Check sheet for the modelled part. Datum: model origin and axes. Units: mm. A direction names the side the tool comes from. Round coordinates to 2 decimals unless told otherwise and drop trailing zeros. Loops run counter-clockwise (first coordinate to the right, second up) from the corner with the lowest first, then second, coordinate; pieces in that order, holes last. Notation, with made-up numbers: (49.25, 27.5) -> (78.25, 27.5) arc R18 cw to (78.25, 36.5) -> close; hole circle Ø7 at (4.5, 61). An arc over 180 degrees is marked (long way). Return JSON: item names as keys, results as strings.
from build123d import *

# Parameters (mm, degrees)
F1_DEPTH        = 5
F2_R            = 22.75
F3_DEPTH        = 1
F5_DEPTH        = 4
F6_DEPTH        = 3
F7_R            = 9
F8_DEPTH        = 4.001
F9_R            = 3
F10_R           = 1
F11_R           = 0.5
F13_D           = 2.75
F13_CBORE_D     = 4.6
F13_CBORE_DEPTH = 2
F14_R           = 1.99999
F15_SIZE        = 0.4
F16_ANGLE       = 180


# Not quite as in the source:
# - a fillet or chamfer is up to 0.001 mm smaller than in the source, because OpenCascade refuses the exact size


with BuildPart() as f1:
    # F0 (on Top) → F1 (new body)
    with BuildSketch(Plane.XY):
        Polygon((23.5, -23.5), (23.5, 23.5), (-23.5, 23.5), (-23.5, 12.5), (-33.5, 12.5), (-33.5, -12.5), (-23.5, -12.5), (-23.5, -23.5), (-12.5, -23.5), (-12.5, -33.5), (12.5, -33.5), (12.5, -23.5), align=None)
    extrude(amount=F1_DEPTH)

    # F2 (on face) → F3 (cut)
    with BuildSketch(Plane(origin=(0, 0, 0), x_dir=(1, 0, 0), z_dir=(0, 0, -1))):
        Circle(F2_R)
    extrude(amount=-F3_DEPTH, mode=Mode.SUBTRACT)

    # F4 (on face) → F5 (join)
    with BuildSketch(Plane.XY):
        with BuildLine():
            ThreePointArc((-16.086679292, -16.086679252), (-20.153889553, -18.8043023144), (-15.3562879116, -17.85))
            ThreePointArc((-15.3562879116, -17.85), (-15.546110447, -16.8956976856), (-16.086679292, -16.086679252))
        make_face()
        with BuildLine():
            ThreePointArc((20.3437120884, 17.85), (16.8956976987, 20.1538895584), (16.086679272, 16.086679272))
            ThreePointArc((16.086679272, 16.086679272), (18.8043023013, 15.5461104416), (20.3437120884, 17.85))
        make_face()
    extrude(amount=-F5_DEPTH)

    # F4 (on face) → F6 (cut)
    with BuildSketch(Plane.XY):
        with BuildLine():
            ThreePointArc((11.5, -19.6293784925), (0, -22.75), (-11.5, -19.6293784925))
            Line((-11.5, -19.6293784925), (-11.5, -32.5))
            Line((-11.5, -32.5), (11.5, -32.5))
            Line((11.5, -32.5), (11.5, -19.6293784925))
        make_face()
        with BuildLine():
            Line((-32.5, -11.5), (-19.6293784925, -11.5))
            ThreePointArc((-19.6293784925, -11.5), (-22.75, 0), (-19.6293784925, 11.5))
            Line((-19.6293784925, 11.5), (-32.5, 11.5))
            Line((-32.5, 11.5), (-32.5, -11.5))
        make_face()
    extrude(amount=F6_DEPTH, mode=Mode.SUBTRACT)

    # F7 (on face) → F8 (cut, through all)
    with BuildSketch(Plane(origin=(0, 0, 1), x_dir=(1, 0, 0), z_dir=(0, 0, -1))):
        Circle(F7_R)
    extrude(amount=-F8_DEPTH, mode=Mode.SUBTRACT)

    # F9
    f9_edges = [f1.edges().sort_by_distance(p)[0] for p in [
        (-23.5, 23.5, 2.5),
        (23.5, 23.5, 2.5),
        (23.5, -23.5, 2.5),
        (-23.5, -23.5, 2.5),
    ]]
    fillet(f9_edges, radius=F9_R)

    # F10
    f10_edges = [f1.edges().sort_by_distance(p)[0] for p in [
        (-32.5, -11.5, 1.5),
        (-33.5, 12.5, 2.5),
        (-32.5, 11.5, 1.5),
        (-33.5, -12.5, 2.5),
        (-12.5, -33.5, 2.5),
        (12.5, -33.5, 2.5),
        (-11.5, -32.5, 1.5),
        (11.5, -32.5, 1.5),
        (-23.5, -12.5, 2.5),
        (-23.5, 12.5, 2.5),
        (-12.5, -23.5, 2.5),
        (12.5, -23.5, 2.5),
        (-19.629378, -11.5, 2),
        (-19.629378, 11.5, 2),
        (11.5, -19.629378, 2),
        (-11.5, -19.629378, 2),
    ]]
    fillet(f10_edges, radius=F10_R)

    # F11
    f11_edges = [f1.edges().sort_by_distance(p)[0] for p in [
        (-19.629378, -11.5, 0.5),
        (-11.5, -19.629378, 0.5),
        (11.5, -19.629378, 0.5),
        (-19.629378, 11.5, 0.5),
    ]]
    fillet(f11_edges, radius=F11_R)

    # F13 (through all)
    with Locations(Plane.XY.offset(5)):
        with Locations((-17.85, -17.85), (17.85, 17.85)):
            CounterBoreHole(F13_D / 2, F13_CBORE_D / 2, F13_CBORE_DEPTH)

    # F14 (radius 2 in the source; OpenCascade refuses exactly that, so slightly less here)
    f14_edges = [f1.edges().sort_by_distance(p)[0] for p in [
        (-9, 0, 5),
        (-9, 0, 1),
    ]]
    fillet(f14_edges, radius=F14_R)

    # F15
    f15_edges = [f1.edges().sort_by_distance(p)[0] for p in [
        (-33.5, 0, 5),
    ]]
    chamfer(f15_edges, length=F15_SIZE)


with BuildPart() as f1_1:
    # F16: moved
    add(f1.part.rotate(Axis((0, -33.5, 0), (-1, 0, 0)), F16_ANGLE))


with BuildPart() as f1_2:
    # F17: moved
    add(f1_1.part.moved(Location((0, 50, 0))))


solid = f1_2.part
Q1. Section check D-D (x = -17.85). Record the boundary of the cut face in (y, z) (3 decimals), then the cut area to 3 significant figures.
Results list:
{"outline": "(-40.5, -4.6) -> (-40.1, -5) -> (-1.45, -5) -> (-1.45, -3) -> (-0.525, -3) -> (-0.525, 4) -> (-1.644, 4) -> (-1.644, 0) -> (-2.895, 0) -> (-2.895, -1) -> (-31.105, -1) -> (-31.105, 0) -> (-40.5, 0) -> close; (2.225, -3) -> (3.15, -3) -> (3.15, -5) -> (6.1, -5) -> (6.5, -4.6) -> (6.5, 0) -> (3.344, 0) -> (3.344, 4) -> (2.225, 4) -> close", "area": "198 mm^2"}
Q2. Go/stop test with flat-tipped pins: pin 1 (2.5 mm diameter, centred on x = -17, y = 1, fed in from -Z); pin 2 (3.5 mm diameter, centred on x = -24, z = -1.5, fed in from -Y); pin 3 (1.5 mm diameter, centred on x = -16.5, y = -28.5, fed in from +Z); pin 4 (7.5 mm diameter, centred on x = -17.85, y = 0.85, fed in from +Z). Record where each tip stops, or that it passes through.
Results list:
{"pin 1": "z = -3", "pin 2": "y = -39.94", "pin 3": "z = -1", "pin 4": "z = 4"}
Q3. Section check C-C (y = 9). Record the boundary of the cut face in (x, z), then the cut area to 3 significant figures.
Results list:
{"outline": "(-12.5, -4.6) -> (-12.1, -5) -> (12.1, -5) -> (12.5, -4.6) -> (12.5, 0) -> (11.5, 0) -> (11.5, -3) -> (-11.5, -3) -> (-11.5, 0) -> (-12.5, 0) -> close", "area": "55.8 mm^2"}
Q4. Material ranges on line 1 (Y direction, x = 17.85, z = 0.25) (3 decimals); line 2 (Y direction, x = -17.85, z = -3.9); line 3 (X direction, y = -14, z = -1.75), recorded low to high.
Results list:
{"line 1": "-37.344 to -36.225, -33.475 to -32.356", "line 2": "-40.5 to -1.45, 3.15 to 6.5", "line 3": "-33.5 to -32.5, -22.55 to -8.95, 8.95 to 23.5"}
Q5. Tool access check on faces 1 (the cylindrical face through (-20.148, 0.749, -4.014)), 2 (the flat face through (17, 6.5, -2)), 3 (the flat face through (-28, -17, -3)). Record the directions out of +Z, -Z, +X, -X, +Y, -Y that give a thin tool (end or side, any length) a straight path to the whole face; none if there is none.
Results list:
{"face 1": "-Z", "face 2": "+Z, -Z, +X, +Y", "face 3": "+Z"}
Q6. Draft check along Y on faces 4 (the cylindrical face through (-22.75, -16.85, -1.99)), 5 (the flat face through (-17, 6.5, -2)), 6 (the cylindrical face through (0.15, 5.75, -1.99)), 7 (the flat face through (-28, -29.5, -2)). Enter one of: released by +Y, released by -Y, zero draft, split by the parting line, or undercut.
Results list:
{"face 4": "undercut", "face 5": "released by +Y", "face 6": "undercut", "face 7": "released by -Y"}
